Verification items for the finished model (mm, model axes). Face numbers are marked on the shaded views. A direction names the side the tool comes from. Round coordinates to 2 decimals unless told otherwise and drop trailing zeros. Loops run counter-clockwise (first coordinate to the right, second up) from the corner with the lowest first, then second, coordinate; pieces in that order, holes last. Notation, with made-up numbers: (1, -32.75) -> (5, -32.75) arc R27 ccw to (5, 5.25) -> close; hole circle Ø2 at (83, 13). An arc over 180 degrees is marked (long way). Write item = value, one per line.
```python
from build123d import *

# Parameters (mm, degrees)
SKETCH_W                = 158.8
SKETCH_H                = 209.8
PAD_DEPTH               = 2
SKETCH001_R             = 2
POCKET_DEPTH            = 528.261316
SKETCH001_MIRRORED_2_R  = 2
POCKET_MIRRORED_2_DEPTH = 528.261316
SKETCH002_W             = 65
SKETCH002_H             = 59
POCKET001_DEPTH         = 2.001
SKETCH003_W             = 65
SKETCH003_H             = 66
PAD001_DEPTH            = 20
POCKET002_DEPTH         = 1.8
SKETCH005_W             = 15
SKETCH005_H             = 59
POCKET003_DEPTH         = 17
SKETCH006_W             = 35
SKETCH006_H             = 59
POCKET004_DEPTH         = 20.001
SKETCH007_W             = 8
SKETCH007_H             = 39
PAD002_DEPTH            = 5


with BuildPart() as part:
    # Sketch → Pad (new body)
    with BuildSketch(Plane.XY):
        Rectangle(SKETCH_W, SKETCH_H)
    extrude(amount=PAD_DEPTH)

    # Sketch001 (on Face6 of Pad) → Pocket (cut, through all)
    with BuildSketch(Plane.XY.offset(2)):
        with Locations((-76.6, 102.1)):
            Circle(SKETCH001_R)
    pocket = extrude(amount=-POCKET_DEPTH, mode=Mode.SUBTRACT)

    # Sketch001 Mirrored 2 → Pocket Mirrored 2 (cut, through all)
    with BuildSketch(Plane(origin=(0, 0, 2), x_dir=(-1, 0, 0), z_dir=(0, 0, -1))):
        with Locations((-76.6, 102.1)):
            Circle(SKETCH001_MIRRORED_2_R)
    pocket_mirrored_2 = extrude(amount=POCKET_MIRRORED_2_DEPTH, mode=Mode.SUBTRACT)

    # Mirrored001: Pocket, Pocket Mirrored 2 across Sketch001 H_Axis
    add(pocket.mirror(Plane(origin=(0, 0, 2), x_dir=(0, 0, 1), z_dir=(0, 1, 0))), mode=Mode.SUBTRACT)
    add(pocket_mirrored_2.mirror(Plane(origin=(0, 0, 2), x_dir=(0, 0, 1), z_dir=(0, 1, 0))), mode=Mode.SUBTRACT)

    # Sketch002 (on Face5 of MultiTransform) → Pocket001 (cut, through all)
    with BuildSketch(Plane.XY.offset(2)):
        with Locations((21.9, -52.4)):
            Rectangle(SKETCH002_W, SKETCH002_H)
    extrude(amount=-POCKET001_DEPTH, mode=Mode.SUBTRACT)

    # Sketch003 (on Face4 of Pocket001) → Pad001 (join)
    with BuildSketch(Plane(origin=(0, 0, 0), x_dir=(1, 0, 0), z_dir=(0, 0, -1))):
        with Locations((21.9, 52.4)):
            Rectangle(SKETCH003_W, SKETCH003_H)
    extrude(amount=PAD001_DEPTH)

    # Sketch004 (on Face5 of Pad001) → Pocket002 (cut)
    with BuildSketch(Plane.XY.offset(2)):
        with BuildLine():
            ThreePointArc((54.4, -60.4), (62.4, -52.4), (54.4, -44.4))
            Line((54.4, -44.4), (54.4, -60.4))
        make_face()
    extrude(amount=-POCKET002_DEPTH, mode=Mode.SUBTRACT)

    # Sketch005 (on Face21 of Pocket002) → Pocket003 (cut)
    with BuildSketch(Plane.XY):
        with Locations((-3.1, -52.4)):
            Rectangle(SKETCH005_W, SKETCH005_H)
        with Locations((46.9, -52.4)):
            Rectangle(SKETCH005_W, SKETCH005_H)
    extrude(amount=-POCKET003_DEPTH, mode=Mode.SUBTRACT)

    # Sketch006 (on Face28 of Pocket003) → Pocket004 (cut, through all)
    with BuildSketch(Plane.XY):
        with Locations((21.9, -52.4)):
            Rectangle(SKETCH006_W, SKETCH006_H)
    extrude(amount=-POCKET004_DEPTH, mode=Mode.SUBTRACT)

    # Sketch007 (on Face4 of Pocket004) → Pad002 (join)
    with BuildSketch(Plane(origin=(0, 0, 0), x_dir=(1, 0, 0), z_dir=(0, 0, -1))):
        with Locations((58.4, 52.4)):
            Rectangle(SKETCH007_W, SKETCH007_H)
    extrude(amount=PAD002_DEPTH)


solid = part.part
```
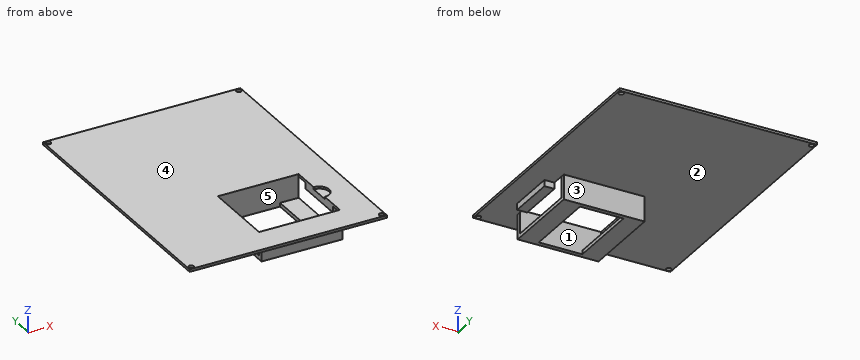
(1) Draft check along Y on the marked faces 1, 2 and 3. Enter one of: released by +Y, released by -Y, zero draft, split by the parting line, or undercut.
Filled sheet:
face_1 = undercut
face_2 = zero draft
face_3 = released by +Y
(2) Material ranges on probe 1 along Y at (x, z) = (76.6, 0.75); probe 2 along Y at (x, z) = (22, -11); probe 3 along Z at (x, y) = (53, 23), recorded low to high. Write a range as from..to.
Filled sheet:
probe_1 = -104.9..-104.1, -100.1..100.1, 104.1..104.9
probe_2 = -85.4..-81.9, -22.9..-19.4
probe_3 = 0..2
(3) Go/stop test with flat-tipped pins: pin 1 Ø4.5 at (x, y) = (-3, -44) entering from +Z; pin 2 Ø9 at (x, y) = (59, -56) entering from +Z; pin 3 Ø6.5 at (x, z) = (7, -6.5) entering from +Y; pin 4 Ø4 at (y, z) = (-47.5, -16.5) entering from +X. Record where each tip stops, or that it passes through.
Filled sheet:
pin_1 = -17
pin_2 = 2
pin_3 = -19.4
pin_4 = 54.4
(4) Sectioned sample at C-C, the plane x = 0. Record the cut outline in (y, z).
Filled sheet:
outline = (-104.9, 0) -> (-85.4, 0) -> (-85.4, -20) -> (-19.4, -20) -> (-19.4, 0) -> (104.9, 0) -> (104.9, 2) -> (-22.9, 2) -> (-22.9, -17) -> (-81.9, -17) -> (-81.9, 2) -> (-104.9, 2) -> close
(5) Sectioned sample at A-A, the plane y = -37. Record the cut outline in (x, z).
Filled sheet:
outline = (-79.4, 0) -> (-10.6, 0) -> (-10.6, 2) -> (-79.4, 2) -> close; (-10.6, -20) -> (4.4, -20) -> (4.4, -17) -> (-10.6, -17) -> close; (39.4, -20) -> (54.4, -20) -> (54.4, -17) -> (39.4, -17) -> close; (54.4, -5) -> (62.4, -5) -> (62.4, 0) -> (79.4, 0) -> (79.4, 2) -> (54.4, 2) -> close
(6) Sectioned sample at D-D, the plane y = 77.5. Record the cut outline in (x, z), and give its area (3 significant figures).
Filled sheet:
outline = (-79.4, 0) -> (79.4, 0) -> (79.4, 2) -> (-79.4, 2) -> close
area = 318 mm2
(7) Sectioned sample at B-B, the plane x = 23.5. Record the cut outline in (y, z), and give its area (3 significant figures).
Filled sheet:
outline = (-104.9, 0) -> (-85.4, 0) -> (-85.4, -20) -> (-81.9, -20) -> (-81.9, 2) -> (-104.9, 2) -> close; (-22.9, -20) -> (-19.4, -20) -> (-19.4, 0) -> (104.9, 0) -> (104.9, 2) -> (-22.9, 2) -> close
area = 442 mm2
(8) Set-up check for the marked faces 4 and 5: record each of +Z, -Z, +X, -X, +Y, -Y from which the full face is reachable in a straight line by a thin tool's end or side.
Filled sheet:
face_4 = +Z, +X, -X, +Y, -Y
face_5 = +Z
